The listing builds one solid part. Answer for the finished solid, in the listing's coordinates (mm). Face numbers are marked on the shaded views. Round coordinates to 2 decimals unless told otherwise and drop trailing zeros. Order: outer loops, then holes, each group sorted by start corner. A loop starts at its lowest first (then second) coordinate and runs counter-clockwise, first axis right, second up. Notation, with made-up numbers: (5.5, -23.75) -> (57.5, -23.75) arc R25 ccw to (57.5, -6.75) -> close; hole circle Ø6 at (5, 43.25). An arc over 180 degrees is marked (long way). Answer in a Markdown table with one row per item. Add a question column.
```python
from build123d import *

# Parameters (mm, degrees)
F0_R     = 5
F1_DEPTH = 25


with BuildPart() as f1:
    # F0 (on Front) → F1 (new body)
    with BuildSketch(Plane.XZ):
        with BuildLine():
            ThreePointArc((0, 15), (4.393398, 4.393398), (15, 0))
            Line((15, 0), (35, 0))
            ThreePointArc((35, 0), (45.606602, 4.393398), (50, 15))
            Line((50, 15), (50, 35))
            ThreePointArc((50, 35), (45.606602, 45.606602), (35, 50))
            ThreePointArc((35, 50), (24.393398, 54.393398), (20, 65))
            ThreePointArc((20, 65), (18.535534, 68.535534), (15, 70))
            Line((15, 70), (5, 70))
            ThreePointArc((5, 70), (1.464466, 68.535534), (0, 65))
            Line((0, 65), (0, 15))
        make_face()
        with Locations((10, 10)):
            Circle(F0_R, mode=Mode.SUBTRACT)
        with Locations((40, 10)):
            Circle(F0_R, mode=Mode.SUBTRACT)
        with Locations((10, 60)):
            Circle(F0_R, mode=Mode.SUBTRACT)
    extrude(amount=F1_DEPTH)


solid = f1.part
```
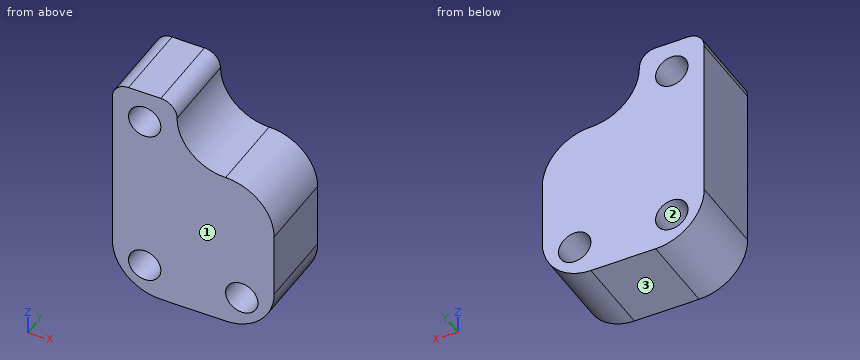
Item 1: Flat-ended cylindrical pins translate along their axes: P1, Ø12, axis at y = -5.5, z = 59, coming from the +X side; P2, Ø6, axis at x = 10, z = 10, coming from the -Y side; P3, Ø1.5, axis at x = 23, y = -15, coming from the +Z side. Find the tip coordinate at first contact, or state that the pin passes through.
Item 2: For a pull along Z with two mould halves and no side action, classify the marked faces 1, 2 and 3 as released by +Z, released by -Z, zero draft, split by the parting line, or undercut.
Item 3: The part is cut by section B-B, the plane x = 10. Give the vertices of the cut face in (y, z).
Item 4: The part is cut by section C-C, the plane y = -12.25. Give the vertices of the cut face in (x, z), and give its area (3 significant figures).
Item 5: The part is cut by section A-A, the plane z = 10. Give the vertices of the cut face in (x, y), and give its area (3 significant figures).
Item 6: Find the intervals of material crossed by probe 1 along Z at (x, y) = (6, -1.5); probe 2 along X at (y, z) = (-8.25, 12.5); probe 3 along Z at (x, y) = (10, -6.5), in increasing order. Write a range as [from, to].
Item 7: The part is cut by section D-D, the plane z = 60. Give the vertices of the cut face in (x, y).
Resolved:
| question | item | result |
|---|---|---|
| 1 | P1 | x = 26 |
| 1 | P2 | through |
| 1 | P3 | z = 57.1 |
| 2 | face 1 | zero draft |
| 2 | face 2 | undercut |
| 2 | face 3 | released by -Z |
| 3 | outline | (-25, 0.86) -> (0, 0.86) -> (0, 5) -> (-25, 5) -> close; (-25, 15) -> (0, 15) -> (0, 55) -> (-25, 55) -> close; (-25, 65) -> (0, 65) -> (0, 70) -> (-25, 70) -> close |
| 4 | outline | (0, 15) arc R15 ccw to (15, 0) -> (35, 0) arc R15 ccw to (50, 15) -> (50, 35) arc R15 ccw to (35, 50) arc R15 cw to (20, 65) arc R5 ccw to (15, 70) -> (5, 70) arc R5 ccw to (0, 65) -> close; hole circle Ø10 at (10, 10); hole circle Ø10 at (10, 60); hole circle Ø10 at (40, 10) |
| 4 | area | 2,560 mm2 |
| 5 | outline | (0.86, -25) -> (5, -25) -> (5, 0) -> (0.86, 0) -> close; (15, -25) -> (35, -25) -> (35, 0) -> (15, 0) -> close; (45, -25) -> (49.14, -25) -> (49.14, 0) -> (45, 0) -> close |
| 5 | area | 707 mm2 |
| 6 | probe 1 | [3, 7], [13, 57], [63, 70] |
| 6 | probe 2 | [0.21, 5.67], [14.33, 35.67], [44.33, 49.79] |
| 6 | probe 3 | [0.86, 5], [15, 55], [65, 70] |
| 7 | outline | (0, -25) -> (5, -25) -> (5, 0) -> (0, 0) -> close; (15, -25) -> (20.86, -25) -> (20.86, 0) -> (15, 0) -> close |
